Verification items for the finished model (mm, model axes). Face numbers are marked on the shaded views. A direction names the side the tool comes from. Give positions to 0.01 mm unless a question says otherwise; leave off trailing zeros. Answer as a JSON object with one key per item and string values.
```python
from build123d import *

# Parameters (mm, degrees)
SKETCH3_R           = 4.35
CUT_EXTRUDE1_DEPTH  = 19.35
SKETCH4_R           = 32
BOSS_EXTRUDE1_DEPTH = 2.5
SKETCH5_R           = 2.555
CUT_EXTRUDE2_DEPTH  = 40
SKETCH6_R           = 20.01
CUT_EXTRUDE3_DEPTH  = 3.7
SKETCH7_R           = 12.725
CUT_EXTRUDE4_DEPTH  = 16.35
SKETCH8_R           = 9.53
CUT_EXTRUDE5_DEPTH  = 16.35
SKETCH9_R           = 2.15
CUT_EXTRUDE6_DEPTH  = 30


with BuildPart() as part:
    # Sketch1 for Loft3 → Loft3 section 0
    with BuildSketch(Plane.XY):
        with BuildLine():
            # circular arc as an exact rational Bezier (weights 1, cos(half-angle), 1)
            Bezier((-22.068965517, 23.172413793), (-22.634146342, 22.634146342), (-23.172413793, 22.068965517), weights=[1, 0.999702691, 1])
            Bezier((-23.172413793, 22.068965517), (-44.190476191, 0), (-23.172413793, -22.068965517), weights=[1, 0.724137931, 1])
            Bezier((-23.172413793, -22.068965517), (-22.634146342, -22.634146342), (-22.068965517, -23.172413793), weights=[1, 0.999702691, 1])
            Bezier((-22.068965517, -23.172413793), (0, -44.190476191), (22.068965517, -23.172413793), weights=[1, 0.724137931, 1])
            Bezier((22.068965517, -23.172413793), (22.634146342, -22.634146342), (23.172413793, -22.068965517), weights=[1, 0.999702691, 1])
            Bezier((23.172413793, -22.068965517), (44.190476191, 0), (23.172413793, 22.068965517), weights=[1, 0.724137931, 1])
            Bezier((23.172413793, 22.068965517), (22.634146342, 22.634146342), (22.068965517, 23.172413793), weights=[1, 0.999702691, 1])
            Bezier((22.068965517, 23.172413793), (0, 44.190476191), (-22.068965517, 23.172413793), weights=[1, 0.724137931, 1])
        make_face()
    # Sketch2 → Loft3 section 1
    with BuildSketch(Plane(origin=(0, 0, -18.85), x_dir=(-1, 0, 0), z_dir=(0, 0, -1))):
        Polygon((20, 21), (21, 20), (21, -20), (20, -21), (-20, -21), (-21, -20), (-21, 20), (-20, 21), align=None)
    loft()

    # Sketch3 → Cut-Extrude1 (cut)
    with BuildSketch(Plane(origin=(0, 0, -18.85), x_dir=(-1, 0, 0), z_dir=(0, 0, -1))):
        with Locations((25.4, 0)):
            Circle(SKETCH3_R)
        with Locations((-25.4, 0)):
            Circle(SKETCH3_R)
    extrude(amount=-CUT_EXTRUDE1_DEPTH, mode=Mode.SUBTRACT)

    # Sketch4 → Boss-Extrude1 (add)
    with BuildSketch(Plane.XY):
        with Locations(Location((0, 0, 0), (0, 0, 136.397181012))):
            Circle(SKETCH4_R)
    extrude(amount=BOSS_EXTRUDE1_DEPTH)

    # Sketch5 → Cut-Extrude2 (cut)
    with BuildSketch(Plane(origin=(0, 0, -18.85), x_dir=(-1, 0, 0), z_dir=(0, 0, -1))):
        with Locations(Location((25.4, 0, 0), (0, 0, 180))):
            Circle(SKETCH5_R)
        with Locations(Location((-25.4, 0, 0), (0, 0, 180))):
            Circle(SKETCH5_R)
    extrude(amount=-CUT_EXTRUDE2_DEPTH, mode=Mode.SUBTRACT)

    # Sketch6 → Cut-Extrude3 (cut)
    with BuildSketch(Plane(origin=(0, 0, -18.85), x_dir=(-1, 0, 0), z_dir=(0, 0, -1))):
        Circle(SKETCH6_R)
    extrude(amount=-CUT_EXTRUDE3_DEPTH, mode=Mode.SUBTRACT)

    # Sketch7 → Cut-Extrude4 (cut)
    with BuildSketch(Plane(origin=(0, 0, -18.85), x_dir=(-1, 0, 0), z_dir=(0, 0, -1))):
        Circle(SKETCH7_R)
    extrude(amount=-CUT_EXTRUDE4_DEPTH, mode=Mode.SUBTRACT)

    # Sketch8 → Cut-Extrude5 (cut)
    with BuildSketch(Plane(origin=(0, 0, -2.5), x_dir=(-1, 0, 0), z_dir=(0, 0, -1))):
        Circle(SKETCH8_R)
    extrude(amount=-CUT_EXTRUDE5_DEPTH, mode=Mode.SUBTRACT)

    # Sketch9 → Cut-Extrude6 (cut)
    with BuildSketch(Plane(origin=(0, 0, -18.85), x_dir=(-1, 0, 0), z_dir=(0, 0, -1))):
        with Locations((-17.960512242, 17.960512242)):
            Circle(SKETCH9_R)
        with Locations(Location((17.960512242, 17.960512242, 0), (0, 0, 180))):
            Circle(SKETCH9_R)
        with Locations(Location((-17.960512242, -17.960512242, 0), (0, 0, 180))):
            Circle(SKETCH9_R)
        with Locations(Location((17.960512242, -17.960512242, 0), (0, 0, 180))):
            Circle(SKETCH9_R)
    extrude(amount=-CUT_EXTRUDE6_DEPTH, mode=Mode.SUBTRACT)


solid = part.part
```
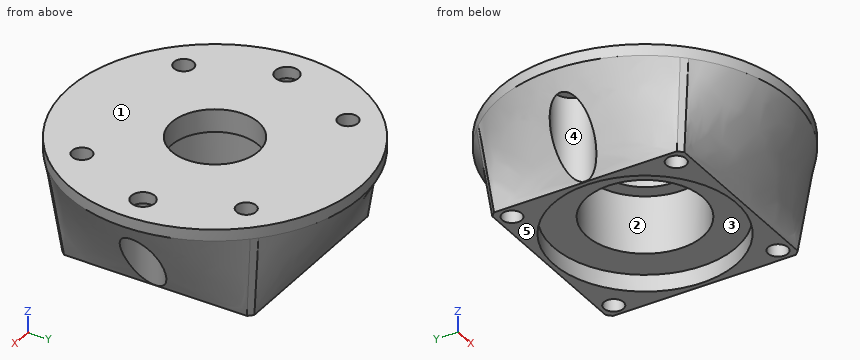
1) Thickness scan on L1, parallel to Y at x = -18, z = 0.25; L2, parallel to X at y = -17, z = -3.5; L3, parallel to X at y = 17.5, z = -13. Record the ranges inside material, lowest first.
Completed:
{"L1": "y = -26.46 to -20.11, -15.81 to 15.81, 20.11 to 26.46", "L2": "x = -25.72 to -19.88, -16.04 to 16.04, 19.88 to 25.72", "L3": "x = -22.42 to -20.06, -15.86 to 15.86, 20.06 to 22.42"}
2) Go/stop test with flat-tipped pins: pin 1 (8 mm diameter, centred on x = -25.4, y = 0, fed in from -Z); pin 2 (4 mm diameter, centred on x = -17.96, y = -17.96, fed in from +Z); pin 3 (4 mm diameter, centred on y = 21.5, z = -14, fed in from -X); pin 4 (2 mm diameter, centred on x = -24, z = -8, fed in from +Y). Record where each tip stops, or that it passes through.
Completed:
{"pin 1": "stops at z = 0", "pin 2": "passes through", "pin 3": "stops at x = -21.89", "pin 4": "stops at y = 19.67"}
3) Release check for a two-part mould opening along Z. For the marked faces 1, 2 and 3 record: pulls with the +Z half, pulls with the -Z half, needs draft (parallel to the pull), parting line crosses it, or undercut.
Completed:
{"face 1": "pulls with the +Z half", "face 2": "needs draft", "face 3": "pulls with the -Z half"}
4) Access from +Z, -Z, +X, -X, +Y, -Y to the whole of each face (thin tool, end or side, straight path). Record for the marked faces 4 and 5.
Completed:
{"face 4": "-Z", "face 5": "-Z, +X, -X, +Y, -Y"}
5) Section check A-A on y = 0. Count the separate pieces of the cut face and the enclosed holes in it, and give its area (3 significant figures).
Completed:
{"separate pieces": "4", "enclosed holes": "0", "area": "371 mm2"}
